CAD build for the part. Positions are in the model's coordinates, mm. Coordinates: 2 decimals unless noted, no trailing zeros. Loops run counter-clockwise (first coordinate to the right, second up) from the corner with the lowest first, then second, coordinate; pieces in that order, holes last. Notation, with made-up numbers: (-17, 84) -> (-10, 84) arc R23 ccw to (-10, 112) -> close; hole circle Ø1 at (-29, -34). An arc over 180 degrees is marked (long way). Write each question's results on one line, items separated by ' | '.
from build123d import *

# Parameters (mm, degrees)
F0_R     = 2.15
F1_DEPTH = 3.2
F3_DEPTH = 74
F4_DEPTH = 32.4


with BuildPart() as f1:
    # F0 (on Top) → F1 (new body)
    with BuildSketch(Plane.XY):
        Polygon((-25, -25), (-25, -50), (25, -50), (25, -25), (8, -22.5), (8, -17.5), (25, -15), (25, 0), (-25, 0), (-25, -15), (-8, -17.5), (-8, -22.5), align=None)
        with Locations((-21.15, -40)):
            Circle(F0_R, mode=Mode.SUBTRACT)
        with Locations((21.15, -40)):
            Circle(F0_R, mode=Mode.SUBTRACT)
        Polygon((-35, 0), (-25, 0), (25, 0), (35, 0), (35, 225), (-35, 225), align=None)
        with Locations((-10, 5)):
            Circle(F0_R, mode=Mode.SUBTRACT)
        with Locations((-10, 30)):
            Circle(F0_R, mode=Mode.SUBTRACT)
        with Locations((10, 5)):
            Circle(F0_R, mode=Mode.SUBTRACT)
        with Locations((10, 30)):
            Circle(F0_R, mode=Mode.SUBTRACT)
        with Locations((-4, 185)):
            Circle(F0_R, mode=Mode.SUBTRACT)
        with Locations((4, 185)):
            Circle(F0_R, mode=Mode.SUBTRACT)
    extrude(amount=F1_DEPTH)

    # F2 (on Top) → F3 (cut)
    with BuildSketch(Plane.XY):
        Polygon((-20, 168), (-20, 200), (20, 200), (20, 168), (31, 157), (31, 225), (-31, 225), (-31, 157), align=None)
        Polygon((-31, 49), (-31, 157), (-31, 225), (-35, 225), (-35, 0), (-31, 0), align=None)
        Polygon((31, 225), (31, 157), (31, 49), (31, 0), (35, 0), (35, 225), align=None)
        Polygon((-16, 35), (-31, 49), (-31, 0), (-16, 0), align=None)
        Polygon((31, 0), (31, 49), (16, 35), (16, 0), align=None)
        Polygon((23, 154.432595), (20.625565, 158), (18, 154.432595), (18, 45), (23, 54.432595), align=None)
        Polygon((-18, 154.432595), (-20.625565, 158), (-23, 154.432595), (-23, 54.432595), (-18, 45), align=None)
    extrude(amount=F3_DEPTH, mode=Mode.SUBTRACT)

    # F2 (on Top) → F4 (cut)
    with BuildSketch(Plane.XY):
        Polygon((-20, 168), (-20, 200), (20, 200), (20, 168), (31, 157), (31, 225), (-31, 225), (-31, 157), align=None)
        Polygon((-31, 49), (-31, 157), (-31, 225), (-35, 225), (-35, 0), (-31, 0), align=None)
        Polygon((31, 225), (31, 157), (31, 49), (31, 0), (35, 0), (35, 225), align=None)
        Polygon((-16, 35), (-31, 49), (-31, 0), (-16, 0), align=None)
        Polygon((31, 0), (31, 49), (16, 35), (16, 0), align=None)
        Polygon((23, 154.432595), (20.625565, 158), (18, 154.432595), (18, 45), (23, 54.432595), align=None)
        Polygon((-18, 154.432595), (-20.625565, 158), (-23, 154.432595), (-23, 54.432595), (-18, 45), align=None)
    extrude(amount=-F4_DEPTH, mode=Mode.SUBTRACT)


solid = f1.part
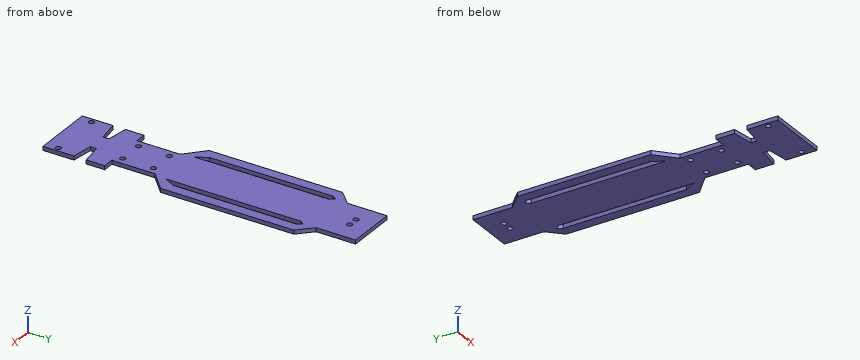
1) Drill centre lines: L1, parallel to X at y = 57.5, z = 2.35; L2, parallel to Y at x = -9, z = 2.7; L3, parallel to X at y = 185, z = 1.65. Where is each one in solid material? Low to high. Write a range as from..to.
Outcome:
L1: x = -31..-23, -18..18, 23..31 | L2: y = -50..-22.65, -17.35..3.1, 6.9..28.1, 31.9..200 | L3: x = -20..-6.15, -1.85..1.85, 6.15..20
2) Slice it at A-A (x = 4). Write the cut outline in (y, z), then the cut area to 3 significant figures.
Outcome:
outline: (-50, 0) -> (182.85, 0) -> (182.85, 3.2) -> (-50, 3.2) -> close; (187.15, 0) -> (200, 0) -> (200, 3.2) -> (187.15, 3.2) -> close | area: 786 mm^2
3) Slice it at C-C (z = 0.7). Count the separate pieces of the cut face and the enclosed holes in it, then the cut area to 3 significant figures.
Outcome:
separate pieces: 1 | enclosed holes: 10 | area: 11,400 mm^2
4) Slice it at B-B (y = -40). Write the cut outline in (x, z).
Outcome:
outline: (-25, 0) -> (-23.3, 0) -> (-23.3, 3.2) -> (-25, 3.2) -> close; (-19, 0) -> (19, 0) -> (19, 3.2) -> (-19, 3.2) -> close; (23.3, 0) -> (25, 0) -> (25, 3.2) -> (23.3, 3.2) -> close
5) Slice it at D-D (y = 104.5). Write the cut outline in (x, z), then the cut area to 3 significant figures.
Outcome:
outline: (-31, 0) -> (-23, 0) -> (-23, 3.2) -> (-31, 3.2) -> close; (-18, 0) -> (18, 0) -> (18, 3.2) -> (-18, 3.2) -> close; (23, 0) -> (31, 0) -> (31, 3.2) -> (23, 3.2) -> close | area: 166 mm^2
6) Pin check, flat tips, straight feed: pin 1 (3.5 mm diameter, centred on x = -21.15, y = -40, fed in from -Z); pin 2 (1.6 mm diameter, centred on y = 183.5, z = 1.5, fed in from -X). Stop position of each tip, or through.
Outcome:
pin 1: passes through | pin 2: stops at x = -20
